Study the drawing (mm; zero at the part's minimum x, y, z) and answer. Give positions to 0.01 mm unless a question says otherwise; leave off trailing zeros. Write each loop counter-clockwise with the first axis right and the second up, starting at its lowest first coordinate (ties: lowest second). Pieces come first, ordered by that corner, then holes.
1) Find section B-B (z = 44.45). Determine the outline of the cut face in (x, y).
2) Find section C-C (y = 60.5). Determine the outline of the cut face in (x, z), plus the area to 3 significant figures.
3) Given pin 1 Ø10 at (x, y) = (50, 21) entering from +Z; pin 2 Ø8 at (y, z) = (61.5, 32) entering from +X; pin 3 Ø6 at (x, y) = (50.5, 80.5) entering from +Z (1 decimal), each flat-ended and moving along its own axis, determine where each tip first touches the part or whether it passes through.
4) Find section D-D (y = 43.5). Determine the outline of the cut face in (x, z).
5) Find section A-A (x = 44.45). Determine the outline of the cut face in (y, z), plus the area to 3 significant figures.
6) Straight lines are drawn through the part: probe 1 along X at (y, z) = (73, 44.45); probe 2 along Z at (x, y) = (35.5, 65.5). For each, find the intervals that lie inside material, in ascending order.
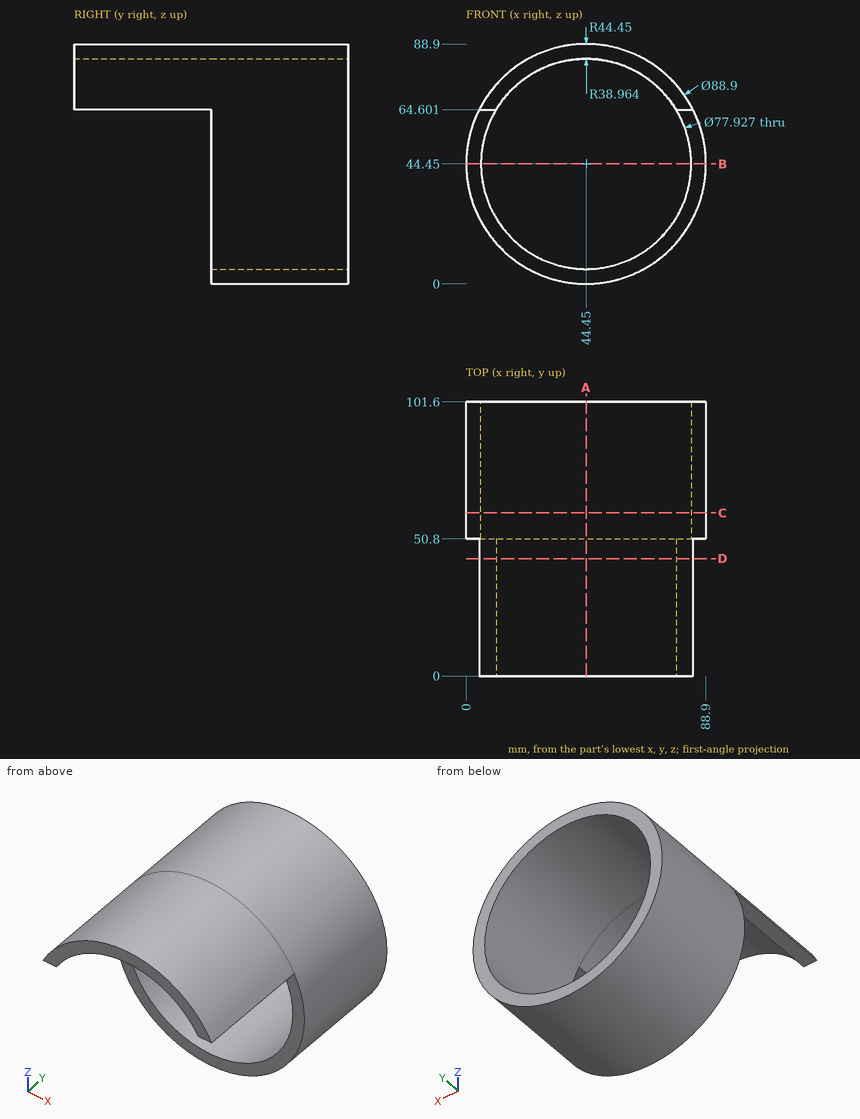
Results:
1. outline: (0, 50.8) - (5.49, 50.8) - (5.49, 101.6) - (0, 101.6) - close; (83.41, 50.8) - (88.9, 50.8) - (88.9, 101.6) - (83.41, 101.6) - close
2. outline: circle Ø88.9 at (44.45, 44.45); hole circle Ø77.93 at (44.45, 44.45)
2. area: 1,440 mm2
3. pin 1: stops at z = 88.9
3. pin 2: stops at x = 88.09
3. pin 3: stops at z = 88.8
4. outline: (4.83, 64.6) - (11.1, 64.6) arc R38.96 cw to (77.8, 64.6) - (84.07, 64.6) arc R44.45 ccw to start
5. outline: (0, 83.41) - (101.6, 83.41) - (101.6, 88.9) - (0, 88.9) - close; (50.8, 0) - (101.6, 0) - (101.6, 5.49) - (50.8, 5.49) - close
5. area: 836 mm2
6. probe 1: x = 0 to 5.49, 83.41 to 88.9
6. probe 2: z = 0.91 to 6.53, 82.37 to 87.99
